from build123d import *

# Parameters (mm, degrees)
RESSALTO_EXTRUS_O1_DEPTH = 12.5
ESBO_O5_R                = 5
RESSALTO_EXTRUS_O2_DEPTH = 1
ESBO_O6_R                = 5
RESSALTO_EXTRUS_O3_DEPTH = 1
ESBO_O2_R                = 2.5
CORTE_EXTRUS_O1_DEPTH    = 49.592694924
ESBO_O3_R                = 2.5
CORTE_EXTRUS_O2_DEPTH    = 49.592694924
ESBO_O7_R                = 5
CORTE_EXTRUS_O3_DEPTH    = 2
ESCALA1_SCALE            = 0.5
CROQUIS4_R               = 5
CORTAR_EXTRUIR3_DEPTH    = 1
CROQUIS9_R               = 2.25
CORTAR_EXTRUIR6_DEPTH    = 24.437416667
CROQUIS10_R              = 2.851109387
CORTAR_EXTRUIR7_DEPTH    = 16
CORTAR_EXTRUIR8_START    = -1
CROQUIS11_R              = 5
CORTAR_EXTRUIR8_DEPTH    = 1
CROQUIS13_R              = 2.5
CROQUIS13_R_2            = 1.25
CORTAR_EXTRUIR9_DEPTH    = 1
CROQUIS12_R              = 3
CROQUIS12_R_2            = 2.25
SALIENTE_EXTRUIR3_DEPTH  = 0.5
REDONDEO1_R              = 0.2
CROQUIS14_R              = 6.25
CROQUIS14_R_2            = 5
SALIENTE_EXTRUIR5_DEPTH  = 2


with BuildPart() as part:
    # Esboço1 → Ressalto-extrusão1 (new, symmetric)
    with BuildSketch(Plane(origin=(0, 0, 0), x_dir=(1, 0, 0), z_dir=(0, 1, 0))):
        with BuildLine():
            Line((-21, -11), (-21, 11))
            ThreePointArc((-21, 11), (-18.071067812, 18.071067812), (-11, 21))
            Line((-11, 21), (11, 21))
            ThreePointArc((11, 21), (18.071067812, 18.071067812), (21, 11))
            Line((21, 11), (21, -11))
            ThreePointArc((21, -11), (18.071067812, -18.071067812), (11, -21))
            Line((11, -21), (-11, -21))
            ThreePointArc((-11, -21), (-18.071067812, -18.071067812), (-21, -11))
        make_face()
        with BuildLine():
            Line((-11, -16), (11, -16))
            ThreePointArc((11, -16), (14.535533906, -14.535533906), (16, -11))
            Line((16, -11), (16, 11))
            ThreePointArc((16, 11), (14.535533906, 14.535533906), (11, 16))
            Line((11, 16), (-11, 16))
            ThreePointArc((-11, 16), (-14.535533906, 14.535533906), (-16, 11))
            Line((-16, 11), (-16, -11))
            ThreePointArc((-16, -11), (-14.535533906, -14.535533906), (-11, -16))
        make_face(mode=Mode.SUBTRACT)
    extrude(amount=RESSALTO_EXTRUS_O1_DEPTH, both=True)

    # Esboço5 → Ressalto-extrusão2 (add)
    with BuildSketch(Plane.XY.offset(-16)):
        Circle(ESBO_O5_R)
    ressalto_extrus_o2 = extrude(amount=RESSALTO_EXTRUS_O2_DEPTH)

    # Espelhar1: Ressalto-extrusão2 across plane
    add(ressalto_extrus_o2.mirror(Plane.XY))

    # Esboço6 → Ressalto-extrusão3 (add)
    with BuildSketch(Plane(origin=(-16, 0, 0), x_dir=(0, 0, -1), z_dir=(1, 0, 0))):
        Circle(ESBO_O6_R)
    ressalto_extrus_o3 = extrude(amount=RESSALTO_EXTRUS_O3_DEPTH)

    # Espelhar2: Ressalto-extrusão3 across plane
    add(ressalto_extrus_o3.mirror(Plane(origin=(0, 0, 0), x_dir=(0, 0, 1), z_dir=(1, 0, 0))))

    # Esboço2 → Corte-extrusão1 (cut, through all)
    with BuildSketch(Plane.XY.offset(21)):
        Circle(ESBO_O2_R)
    extrude(amount=-CORTE_EXTRUS_O1_DEPTH, mode=Mode.SUBTRACT)

    # Esboço3 → Corte-extrusão2 (cut, through all)
    with BuildSketch(Plane.ZY.offset(21)):
        Circle(ESBO_O3_R)
    extrude(amount=-CORTE_EXTRUS_O2_DEPTH, mode=Mode.SUBTRACT)

    # Esboço7 → Corte-extrusão3 (cut)
    with BuildSketch(Plane(origin=(21, 0, 0), x_dir=(0, 0, -1), z_dir=(1, 0, 0))):
        Circle(ESBO_O7_R)
    corte_extrus_o3 = extrude(amount=-CORTE_EXTRUS_O3_DEPTH, mode=Mode.SUBTRACT)

    # Espelhar3: Corte-extrusão3 across plane
    add(corte_extrus_o3.mirror(Plane(origin=(0, 0, 0), x_dir=(0, 0, 1), z_dir=(1, 0, 0))), mode=Mode.SUBTRACT)


with BuildPart() as part_1:
    # Escala1: scaled about (0, 0, 0)
    add(part.part.scale(ESCALA1_SCALE))

    # Croquis4 → Cortar-Extruir3 (cut)
    with BuildSketch(Plane.ZY.offset(10.5)):
        Circle(CROQUIS4_R)
    extrude(amount=-CORTAR_EXTRUIR3_DEPTH, mode=Mode.SUBTRACT)

    # Croquis9 → Cortar-Extruir6 (cut, through all)
    with BuildSketch(Plane.ZY.offset(9.5)):
        Circle(CROQUIS9_R)
    extrude(amount=-CORTAR_EXTRUIR6_DEPTH, mode=Mode.SUBTRACT)

    # Croquis10 → Cortar-Extruir7 (cut)
    with BuildSketch(Plane.ZY.offset(-8)):
        Circle(CROQUIS10_R)
    extrude(amount=CORTAR_EXTRUIR7_DEPTH, mode=Mode.SUBTRACT)

    # Croquis11 → Cortar-Extruir8 (cut)
    with BuildSketch(Plane(origin=(10.5, 0, 0), x_dir=(0, 0, -1), z_dir=(1, 0, 0)).offset(CORTAR_EXTRUIR8_START)):
        with Locations(Location((0, 0, 0), (0, 0, 180))):
            Circle(CROQUIS11_R)
    extrude(amount=CORTAR_EXTRUIR8_DEPTH, mode=Mode.SUBTRACT)

    # Croquis13 → Cortar-Extruir9 (cut)
    with BuildSketch(Plane.XY.offset(10.5)):
        Circle(CROQUIS13_R)
        Circle(CROQUIS13_R_2, mode=Mode.SUBTRACT)
    cortar_extruir9 = extrude(amount=-CORTAR_EXTRUIR9_DEPTH, mode=Mode.SUBTRACT)

    # Simetría4: Cortar-Extruir9 across plane
    add(cortar_extruir9.mirror(Plane.XY), mode=Mode.SUBTRACT)

    # Croquis12 → Saliente-Extruir3 (add)
    with BuildSketch(Plane(origin=(-8, 0, 0), x_dir=(0, 0, -1), z_dir=(1, 0, 0))):
        Circle(CROQUIS12_R)
        with Locations(Location((0, 0, 0), (0, 0, 180))):
            Circle(CROQUIS12_R_2, mode=Mode.SUBTRACT)
    saliente_extruir3 = extrude(amount=SALIENTE_EXTRUIR3_DEPTH)

    # Simetría5: Saliente-Extruir3 across plane
    add(saliente_extruir3.mirror(Plane(origin=(0, 0, 0), x_dir=(0, 0, 1), z_dir=(1, 0, 0))))

    # Redondeo1
    redondeo1_edges = [part_1.edges().sort_by_distance(p)[0] for p in [
        (-8, 0, 3),
        (8, 0, 3),
        (-2.5, 0, -8),
        (-2.5, 0, 8),
    ]]
    fillet(redondeo1_edges, radius=REDONDEO1_R)

    # Croquis14 → Saliente-Extruir5 (add)
    with BuildSketch(Plane(origin=(10.5, 0, 0), x_dir=(0, 0, -1), z_dir=(1, 0, 0))):
        with Locations(Location((0, 0, 0), (0, 0, 151.642363424))):
            Circle(CROQUIS14_R)
        with Locations(Location((0, 0, 0), (0, 0, 180))):
            Circle(CROQUIS14_R_2, mode=Mode.SUBTRACT)
    extrude(amount=SALIENTE_EXTRUIR5_DEPTH)


solid = part_1.part
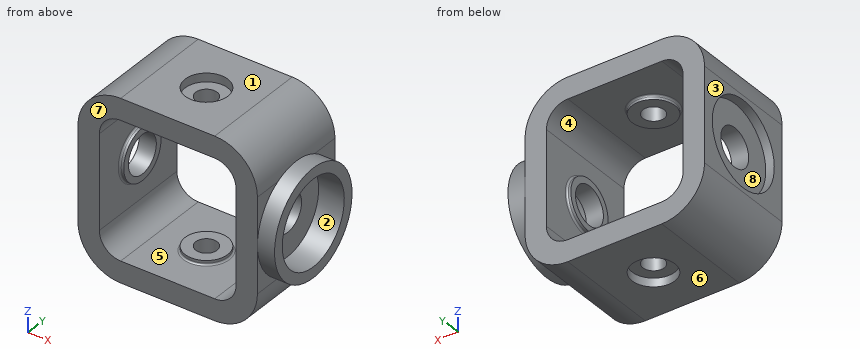
Part model, mm, in its own coordinate system. Face numbers are marked on the shaded views. A direction names the side the tool comes from. Coordinates: 2 decimals unless noted, no trailing zeros. Write each loop counter-clockwise with the first axis right and the second up, starting at its lowest first coordinate (ties: lowest second). Pieces come first, ordered by that corner, then holes. Notation, with made-up numbers: M 71.25,-12 L 119.25,-12 A26 cw 119.25,22 Z; hole C 88.5,87 d7. An arc over 180 degrees is marked long. Return JSON: item names as keys, results as strings.
1. Pull direction Z, two halves, no side cores. Call the marked faces 6, 7 and 8: pulls with the +Z half, pulls with the -Z half, needs draft (parallel to the pull), parting line crosses it, or undercut.
Determined:
{"face 6": "pulls with the -Z half", "face 7": "needs draft", "face 8": "undercut"}
2. Flat gauge pins, fed straight in: pin 1 Ø5 at (y, z) = (0, -1) entering from -X; pin 2 Ø3 at (y, z) = (4, -7) entering from +X; pin 3 Ø1.5 at (x, y) = (-1, -1) entering from +Z; pin 4 Ø2 at (x, y) = (0, 0) entering from +Z. Where does each tip first touch, or does it go through?
Determined:
{"pin 1": "x = -9.5", "pin 2": "x = 10.5", "pin 3": "z = 9.5", "pin 4": "through"}
3. Saw through at D-D, the plane y = 0. Count the separate pieces of the cut face and the enclosed holes in it, then the cut area to 3 significant figures.
Determined:
{"separate pieces": "4", "enclosed holes": "0", "area": "127 mm²"}
4. Saw through at A-A, the plane y = -4.5. Write the cut outline in (x, z), then the cut area to 3 significant figures.
Determined:
{"outline": "M -10.5,-5.5 A5 ccw -5.5,-10.5 L 5.5,-10.5 A5 ccw 10.5,-5.5 L 10.5,-4.34 L 12.5,-4.34 L 12.5,-2.18 L 9.5,-2.18 L 9.5,2.18 L 12.5,2.18 L 12.5,4.34 L 10.5,4.34 L 10.5,5.5 A5 ccw 5.5,10.5 L -5.5,10.5 A5 ccw -10.5,5.5 L -10.5,2.18 L -9.5,2.18 L -9.5,-2.18 L -10.5,-2.18 Z; hole M -8,-5.5 A2.5 ccw -5.5,-8 L 5.5,-8 A2.5 ccw 8,-5.5 L 8,5.5 A2.5 ccw 5.5,8 L -5.5,8 A2.5 ccw -8,5.5 Z", "area": "169 mm²"}
5. Saw through at B-B, the plane z = -3.5. Write the cut outline in (x, y).
Determined:
{"outline": "M -10.5,-6.25 L -8,-6.25 L -8,6.25 L -10.5,6.25 L -10.5,3.57 L -9.5,3.57 L -9.5,-3.57 L -10.5,-3.57 Z; M 8,-6.25 L 10.5,-6.25 L 10.5,-5.18 L 12.5,-5.18 L 12.5,-3.57 L 9.5,-3.57 L 9.5,3.57 L 12.5,3.57 L 12.5,5.18 L 10.5,5.18 L 10.5,6.25 L 8,6.25 Z"}
6. Probe L1, parallel to Z at x = -3.75, y = 0; L2, parallel to Y at x = 11.1, z = 0; L3, parallel to X at y = -1.5, z = -4. List the from-to ranges inside material, lowest first.
Determined:
{"L1": "-10.5 to -8, 8 to 10.5", "L2": "-6.25 to -5, 5 to 6.25", "L3": "-9.5 to -8, 8 to 9.5"}
7. 3-axis set-ups, long thin cutter, end or side, ignore diameter. For the marked faces 1, 2, 3, 4 and 5: which of +Z, -Z, +X, -X, +Y, -Y reach the whole face in a straight line?
Determined:
{"face 1": "+Z, +X, -X, +Y, -Y", "face 2": "+X", "face 3": "+Z, -Z, -X, +Y, -Y", "face 4": "+Y, -Y", "face 5": "none"}
8. Saw through at C-C, the plane x = 10. Write the cut outline in (y, z), then the cut area to 3 significant figures.
Determined:
{"outline": "M -6.25,-7.68 L 6.25,-7.68 L 6.25,7.68 L -6.25,7.68 Z; hole C 0,0 d10", "area": "113 mm²"}
